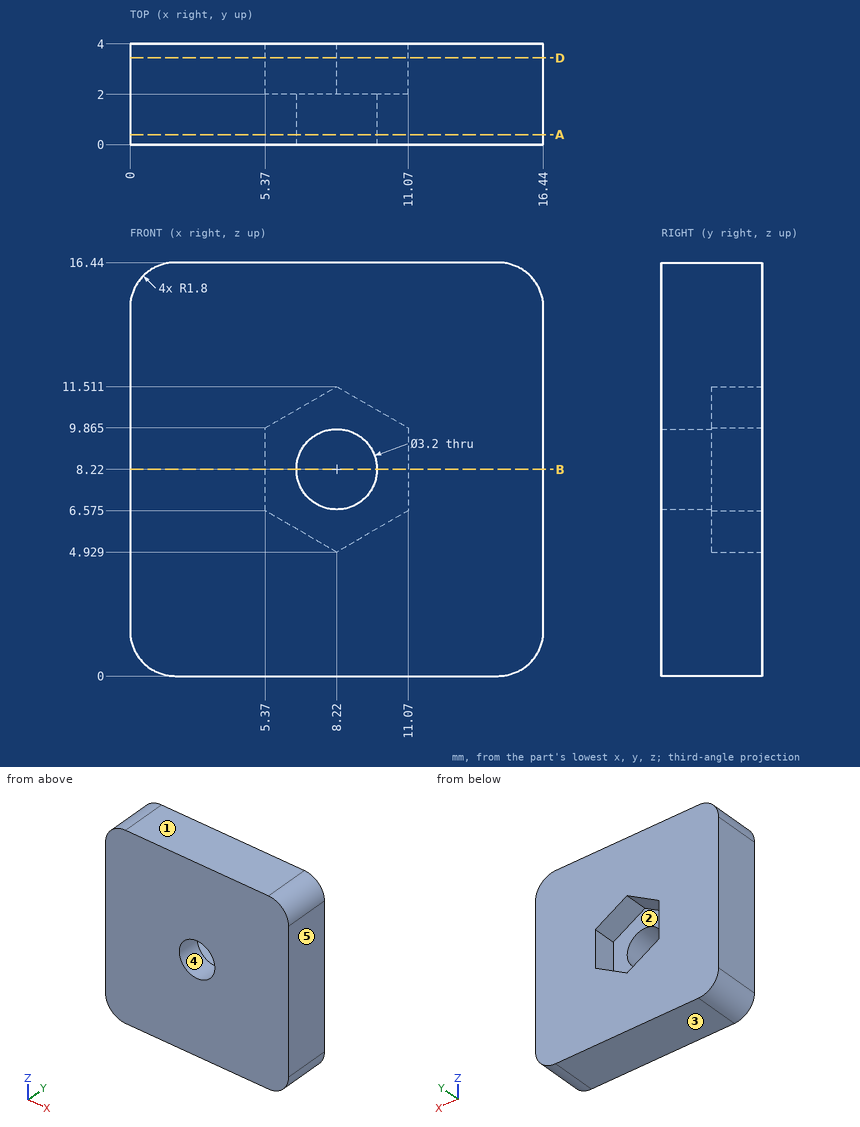
Drawing for the job (mm, zero at the part's lowest x, y, z). A direction names the side the tool comes from. Round coordinates to 2 decimals unless told otherwise and drop trailing zeros. Order: outer loops, then holes, each group sorted by start corner. A loop starts at its lowest first (then second) coordinate and runs counter-clockwise, first axis right, second up. Notation, with made-up numbers: (63, 37.5) -> (76, 37.5) arc R28 cw to (76, 73.5) -> close; hole circle Ø6 at (37, 45). An arc over 180 degrees is marked (long way). Write item = value, one per line. Start each with the question number.
(1) Pull direction X, two halves, no side cores. Call the marked faces 3, 4 and 5: released by +X, released by -X, zero draft, split by the parting line, or undercut.
(2) Cut at A-A, the plane y = 0.4. List the corners of the cut face in (x, z).
(3) Pin check, flat tips, straight feed: P1, Ø1, axis at x = 3, z = 11, coming from the -Y side; P2, Ø1.7, axis at x = 9.5, z = 9, coming from the +Y side. Stop position of each tip, or through.
(4) Cut at B-B, the plane z = 8.22. List the corners of the cut face in (x, y).
(5) Probe line 1 (X direction, y = 0.95, z = 8.22); line 2 (X direction, y = 2.5, z = 6.75); line 3 (Y direction, x = 10, z = 8.25). List the from-to ranges inside material, lowest first. Write a range as [from, to].
(6) Which spindle directions (+Z, -Z, +X, -X, +Y, -Y) get a long thin tool onto all of the face, cutting with end or side? Do the marked faces 1 and 2. Say none if no direction does.
(7) Cut at D-D, the plane y = 3.45. List the corners of the cut face in (x, z) (1 decimal).
Model answer:
q1.face_3 = zero draft
q1.face_4 = undercut
q1.face_5 = released by +X
q2.outline = (0, 1.8) arc R1.8 ccw to (1.8, 0) -> (14.64, 0) arc R1.8 ccw to (16.44, 1.8) -> (16.44, 14.64) arc R1.8 ccw to (14.64, 16.44) -> (1.8, 16.44) arc R1.8 ccw to (0, 14.64) -> close; hole circle Ø3.2 at (8.22, 8.22)
q3.P1 = 0
q3.P2 = 2
q4.outline = (0, 0) -> (6.62, 0) -> (6.62, 2) -> (5.37, 2) -> (5.37, 4) -> (0, 4) -> close; (9.82, 0) -> (16.44, 0) -> (16.44, 4) -> (11.07, 4) -> (11.07, 2) -> (9.82, 2) -> close
q5.line_1 = [0, 6.62], [9.82, 16.44]
q5.line_2 = [0, 5.37], [11.07, 16.44]
q5.line_3 = [0, 2]
q6.face_1 = +Z, +X, -X, +Y, -Y
q6.face_2 = +Y
q7.outline = (0, 1.8) arc R1.8 ccw to (1.8, 0) -> (14.6, 0) arc R1.8 ccw to (16.4, 1.8) -> (16.4, 14.6) arc R1.8 ccw to (14.6, 16.4) -> (1.8, 16.4) arc R1.8 ccw to (0, 14.6) -> close; hole (5.4, 6.6) -> (8.2, 4.9) -> (11.1, 6.6) -> (11.1, 9.9) -> (8.2, 11.5) -> (5.4, 9.9) -> close
